Geometry check sheet. Reference: the model listing, model coordinates, mm. Face numbers are marked on the shaded views. A direction names the side the tool comes from. Give positions to 0.01 mm unless a question says otherwise; leave off trailing zeros. Order: outer loops, then holes, each group sorted by start corner. A loop starts at its lowest first (then second) coordinate and runs counter-clockwise, first axis right, second up. Notation, with made-up numbers: M 33,9.5 L 56,9.5 A18 ccw 56,30.5 Z; hole C 40,-39 d5. An arc over 180 degrees is marked long. Answer as CSV lines item,"result". Start each with the question number.
Q1. Section check C-C, the plane z = -77. Record the boundary of the cut face in (x, y), then the cut area to 3 significant figures.
Q2. Mould release check, pull along Y, two halves, no side actions. Record for the marked faces 1, 2, 3 and 4: +Y half, -Y half, draft (parallel to the pull), parting line (faces both ways), or undercut.
Q3. Section check B-B, the plane y = 0. Record the boundary of the cut face in (x, z), then the cut area to 3 significant figures.
Q4. Section check A-A, the plane x = 0. Record the boundary of the cut face in (y, z), then the cut area to 3 significant figures.
Q5. Go/stop test with flat-tipped pins: pin 1 (1.5 mm diameter, centred on y = 33.5, z = -67, fed in from -X); pin 2 (3 mm diameter, centred on y = -32, z = -59, fed in from -X); pin 3 (1.5 mm diameter, centred on x = -13, z = -89, fed in from -Y). Record where each tip stops, or that it passes through.
Q6. Thickness scan on line 1 (X direction, y = 0, z = -91); line 2 (Z direction, x = -13, y = -1). Record the ranges inside material, lowest first.
Q7. Section check D-D, the plane z = 11. Record the boundary of the cut face in (x, y), then the cut area to 3 significant figures.
Q8. Set-up check for the marked faces 5, 6 and 7: record each of +Z, -Z, +X, -X, +Y, -Y from which the full face is reachable in a straight line by a thin tool's end or side.
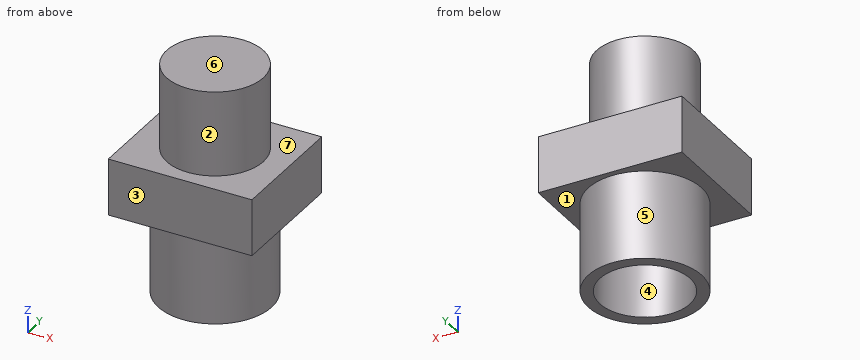
```python
from build123d import *

# Parameters (mm, degrees)
F0_W     = 129.07374
F0_H     = 111.796118
F1_DEPTH = 50.813455
F2_R     = 43.46422
F3_DEPTH = 76.2
F4_R     = 50.947819
F4_R_2   = 40.53744
F5_DEPTH = 79.245634


with BuildPart() as f1:
    # F0 (on Top) → F1 (new body)
    with BuildSketch(Plane.XY):
        Rectangle(F0_W, F0_H)
    extrude(amount=-F1_DEPTH)

    # F2 (on face) → F3 (join)
    with BuildSketch(Plane.XY):
        Circle(F2_R)
    extrude(amount=F3_DEPTH)

    # F4 (on face) → F5 (join)
    with BuildSketch(Plane(origin=(0, 0, -50.813455), x_dir=(1, 0, 0), z_dir=(0, 0, -1))):
        Circle(F4_R)
        Circle(F4_R_2, mode=Mode.SUBTRACT)
    extrude(amount=F5_DEPTH)


solid = f1.part
```
Answer block:
1,outline,"C 0,0 d101.9; hole C 0,0 d81.07"
1,area,"2,990 mm2"
2,face 1,"draft"
2,face 2,"parting line"
2,face 3,"-Y half"
2,face 4,"undercut"
3,outline,"M -64.54,-50.81 L -50.95,-50.81 L -50.95,-130.06 L -40.54,-130.06 L -40.54,-50.81 L 40.54,-50.81 L 40.54,-130.06 L 50.95,-130.06 L 50.95,-50.81 L 64.54,-50.81 L 64.54,0 L 43.46,0 L 43.46,76.2 L -43.46,76.2 L -43.46,0 L -64.54,0 Z"
3,area,"14,800 mm2"
4,outline,"M -55.9,-50.81 L -50.95,-50.81 L -50.95,-130.06 L -40.54,-130.06 L -40.54,-50.81 L 40.54,-50.81 L 40.54,-130.06 L 50.95,-130.06 L 50.95,-50.81 L 55.9,-50.81 L 55.9,0 L 43.46,0 L 43.46,76.2 L -43.46,76.2 L -43.46,0 L -55.9,0 Z"
4,area,"14,000 mm2"
5,pin 1,"stops at x = -39.03"
5,pin 2,"stops at x = -40.81"
5,pin 3,"stops at y = -49.45"
6,line 1,"x = -50.95 to -40.54, 40.54 to 50.95"
6,line 2,"z = -50.81 to 76.2"
7,outline,"C 0,0 d86.93"
7,area,"5,930 mm2"
8,face 5,"-Z"
8,face 6,"+Z, +X, -X, +Y, -Y"
8,face 7,"+Z"
